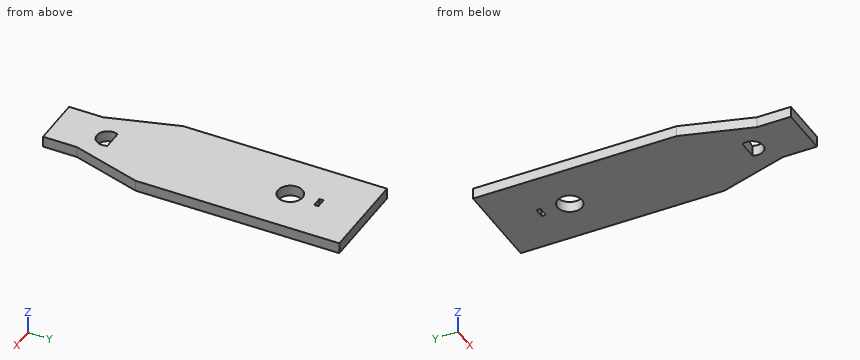
```python
from build123d import *

# Parameters (mm, degrees)
SKETCH1_R           = 3.375
BOSS_EXTRUDE3_DEPTH = 3
SKETCH5_W           = 2.76
SKETCH5_H           = 1.15
CUT_EXTRUDE3_DEPTH  = 448.473185448


with BuildPart() as part:
    # Sketch1 → Boss-Extrude3 (new body)
    with BuildSketch(Plane.XY):
        Polygon((-364.123724325, 176.492478394), (-369.858869661, 195.576225703), (-369.858869661, 251.55599422), (-344.532032114, 251.55599422), (-344.532032114, 195.576225703), (-350.26717745, 176.492478394), (-350.26717745, 167.153932289), (-364.123724325, 167.153932289), align=None)
        with Locations((-357.117541936, 231.55599422)):
            Circle(SKETCH1_R, mode=Mode.SUBTRACT)
    extrude(amount=BOSS_EXTRUDE3_DEPTH)

    # Sketch5 → Cut-Extrude3 (cut, through all)
    with BuildSketch(Plane.XY.offset(-9.5)):
        with BuildLine():
            Line((-359.5563, 182.840556402), (-354.1563, 182.840556402))
            ThreePointArc((-354.1563, 182.840556402), (-356.8563, 178.555993811), (-359.5563, 182.840556402))
        make_face()
        with Locations((-357.117541936, 239.434089807)):
            Rectangle(SKETCH5_W, SKETCH5_H)
    extrude(amount=CUT_EXTRUDE3_DEPTH, mode=Mode.SUBTRACT)


solid = part.part
```
Part model, mm, in its own coordinate system. Round coordinates to 2 decimals unless told otherwise and drop trailing zeros. Write each loop counter-clockwise with the first axis right and the second up, starting at its lowest first coordinate (ties: lowest second). Pieces come first, ordered by that corner, then holes. Notation, with made-up numbers: M 24,42.25 L 50,42.25 A23 ccw 50,67.25 Z; hole C 16,-10 d5. An arc over 180 degrees is marked long. One line per question, with ' | ' between items.
(1) Saw through at A-A on z = 1.4. Write the cut outline in (x, y) (3 decimals).
Answer key:
outline: M -369.859,195.576 L -364.124,176.492 L -364.124,167.154 L -350.267,167.154 L -350.267,176.492 L -344.532,195.576 L -344.532,251.556 L -369.859,251.556 Z; hole C -357.118,231.556 d6.75; hole M -359.556,182.841 A2.993 ccw long -354.156,182.841 Z; hole M -358.498,238.859 L -355.738,238.859 L -355.738,240.009 L -358.498,240.009 Z
(2) Pin check, flat tips, straight feed: pin 1 (6 mm diameter, centred on x = -357.12, y = 231.56, fed in from -Z); pin 2 (0.9 mm diameter, centred on y = 172.5, z = 1, fed in from +X); pin 3 (12 mm diameter, centred on x = -360, y = 180, fed in from -Z); pin 4 (1.5 mm diameter, centred on y = 170, z = 2, fed in from -X). Stop position of each tip, or through.
Answer key:
pin 1: passes through | pin 2: stops at x = -350.27 | pin 3: stops at z = 0 | pin 4: stops at x = -364.12
(3) Probe line 1 along X through (y, z) = (229, 2.35); line 2 along X through (y, z) = (229.5, 1.25); line 3 along X through (y, z) = (190.5, 1.05). List the from-to ranges inside material, lowest first.
Answer key:
line 1: x = -369.86 to -359.32, -354.91 to -344.53 | line 2: x = -369.86 to -359.79, -354.44 to -344.53 | line 3: x = -368.33 to -346.06
(4) Saw through at D-D on y = 192. Write the cut outline in (x, z).
Answer key:
outline: M -368.78,0 L -345.61,0 L -345.61,3 L -368.78,3 Z
(5) Saw through at C-C on x = -366.75. Write the cut outline in (y, z), then the cut area to 3 significant figures.
Answer key:
outline: M 185.23,0 L 251.56,0 L 251.56,3 L 185.23,3 Z | area: 199 mm^2
(6) Saw through at B-B on y = 234. Write the cut outline in (x, z), then the cut area to 3 significant figures.
Answer key:
outline: M -369.86,0 L -359.45,0 L -359.45,3 L -369.86,3 Z; M -354.79,0 L -344.53,0 L -344.53,3 L -354.79,3 Z | area: 62.0 mm^2
